Geometry check sheet. Reference: the model listing, model coordinates, mm. A direction names the side the tool comes from. Give positions to 0.01 mm unless a question says otherwise; leave off trailing zeros. Loops run counter-clockwise (first coordinate to the right, second up) from the corner with the lowest first, then second, coordinate; pieces in that order, holes last. Notation, with made-up numbers: (40, -22) -> (73, -22) arc R28 ccw to (73, 13) -> close; hole circle Ø9 at (70.25, 42.25). An arc over 180 degrees is marked (long way). Answer as a JSON object with one key per item and string values.
from build123d import *

# Parameters (mm, degrees)
F1_DEPTH = 609.6


with BuildPart() as f1:
    # F0 (on Front) → F1 (new body)
    with BuildSketch(Plane.XZ):
        with BuildLine():
            Line((0, 431.8), (0, 0))
            Line((0, 0), (76.2, 0))
            Line((76.2, 0), (76.2, 431.8))
            ThreePointArc((76.2, 431.8), (91.078976, 467.721024), (127, 482.6))
            ThreePointArc((127, 482.6), (162.921024, 467.721024), (177.8, 431.8))
            Line((177.8, 431.8), (177.8, 0))
            Line((177.8, 0), (279.4, 0))
            Line((279.4, 0), (279.4, 327.887458))
            ThreePointArc((279.4, 327.887458), (294.278976, 363.808483), (330.2, 378.687458))
            ThreePointArc((330.2, 378.687458), (366.121024, 363.808483), (381, 327.887458))
            Line((381, 327.887458), (381, 0))
            Line((381, 0), (457.2, 0))
            Line((457.2, 0), (457.2, 565.605909))
            Line((457.2, 565.605909), (381, 565.605909))
            Line((381, 565.605909), (381, 473.937458))
            ThreePointArc((381, 473.937458), (373.560512, 455.976946), (355.6, 448.537458))
            Line((355.6, 448.537458), (304.8, 448.537458))
            ThreePointArc((304.8, 448.537458), (286.839488, 455.976946), (279.4, 473.937458))
            Line((279.4, 473.937458), (279.4, 564.986005))
            Line((279.4, 564.986005), (177.8, 564.986005))
            Line((177.8, 564.986005), (177.8, 533.4))
            ThreePointArc((177.8, 533.4), (170.360512, 515.439488), (152.4, 508))
            Line((152.4, 508), (101.6, 508))
            ThreePointArc((101.6, 508), (83.639488, 515.439488), (76.2, 533.4))
            Line((76.2, 533.4), (76.2, 565.605909))
            Line((76.2, 565.605909), (0, 565.605909))
            Line((0, 565.605909), (0, 431.8))
        make_face()
    extrude(amount=F1_DEPTH)


solid = f1.part
1) Depth check by flat-ended pin: P1, Ø10, axis at x = 124.5, y = -101.5, coming from the +Z side; P2, Ø16, axis at y = -225, z = 554, coming from the -X side; P3, Ø1, axis at x = 204.5, y = -329.5, coming from the +Z side; P4, Ø10, axis at x = 155.5, y = -71, coming from the -Z side. Enter the tip coordinate at first touch or a pass-through.
Geometry check:
{"P1": "stops at z = 508", "P2": "stops at x = 0", "P3": "stops at z = 564.99", "P4": "stops at z = 469.99"}
2) Section check C-C on z = 360.5. Record the cut outline in (x, y), plus the area to 3 significant figures.
Geometry check:
{"outline": "(0, -609.6) -> (76.2, -609.6) -> (76.2, 0) -> (0, 0) -> close; (177.8, -609.6) -> (291.25, -609.6) -> (291.25, 0) -> (177.8, 0) -> close; (369.15, -609.6) -> (457.2, -609.6) -> (457.2, 0) -> (369.15, 0) -> close", "area": "169,000 mm2"}
3) Section check B-B on y = -530. Record the cut outline in (x, z), plus the area to 3 significant figures.
Geometry check:
{"outline": "(0, 0) -> (76.2, 0) -> (76.2, 431.8) arc R50.8 cw to (127, 482.6) arc R50.8 cw to (177.8, 431.8) -> (177.8, 0) -> (279.4, 0) -> (279.4, 327.89) arc R50.8 cw to (381, 327.89) -> (381, 0) -> (457.2, 0) -> (457.2, 565.61) -> (381, 565.61) -> (381, 473.94) arc R25.4 cw to (355.6, 448.54) -> (304.8, 448.54) arc R25.4 cw to (279.4, 473.94) -> (279.4, 564.99) -> (177.8, 564.99) -> (177.8, 533.4) arc R25.4 cw to (152.4, 508) -> (101.6, 508) arc R25.4 cw to (76.2, 533.4) -> (76.2, 565.61) -> (0, 565.61) -> close", "area": "156,000 mm2"}
4) Tool access check on faces 1 (the face through (225, -609.6, 287)), 2 (the face through (170.56, -300.53, 515.64)), 3 (the face through (177.8, -301, 219)). Record the directions out of +Z, -Z, +X, -X, +Y, -Y that give a thin tool (end or side, any length) a straight path to the whole face; none if there is none.
Geometry check:
{"face 1": "+Z, -Z, +X, -X, -Y", "face 2": "+Z, +Y, -Y", "face 3": "-Z, +Y, -Y"}
5) Section check A-A on z = 118. Record the cut outline in (x, y), plus the area to 3 significant figures.
Geometry check:
{"outline": "(0, -609.6) -> (76.2, -609.6) -> (76.2, 0) -> (0, 0) -> close; (177.8, -609.6) -> (279.4, -609.6) -> (279.4, 0) -> (177.8, 0) -> close; (381, -609.6) -> (457.2, -609.6) -> (457.2, 0) -> (381, 0) -> close", "area": "155,000 mm2"}
6) Material ranges on line 1 along X through (y, z) = (-234.5, 49); line 2 along X through (y, z) = (-38, 385); line 3 along X through (y, z) = (-525, 464.5), recorded low to high. Write a range as from..to.
Geometry check:
{"line 1": "x = 0..76.2, 177.8..279.4, 381..457.2", "line 2": "x = 0..76.2, 177.8..457.2", "line 3": "x = 0..88.12, 165.88..281.22, 379.18..457.2"}
